Verification items for the finished model (mm, model axes). A direction names the side the tool comes from. Coordinates: 2 decimals unless noted, no trailing zeros. Order: outer loops, then holes, each group sorted by start corner. A loop starts at its lowest first (then second) coordinate and runs counter-clockwise, first axis right, second up. Notation, with made-up numbers: M 69,69 L 116,69 A21 cw 116,84 Z; hole C -26.5,70.25 d6. An arc over 180 degrees is marked long. Return JSON: item names as keys, results as strings. Group by question number.
Q1. Section check B-B, the plane x = 0. Enter the section's corners in (y, z).
Q2. Thickness scan on probe 1 along Z at (x, y) = (0, 26.5); probe 2 along Z at (x, y) = (-0.25, 63.5); probe 3 along Y at (x, z) = (3.25, 5.5). Record the ranges inside material, lowest first.
Q3. Section check D-D, the plane y = 60. Enter the section's corners in (x, z).
Q4. Section check A-A, the plane z = 0. Enter the section's corners in (x, y), then the cut area to 3 significant figures.
Q5. Mould release check, pull along X, two halves, no side actions. Record for faces 3 (the face through (0, 50.8, 0)), 4 (the face through (-2.87, 25.04, 2.64)), 5 (the face through (-1.65, 68.6, 7.44)), 6 (the face through (0, 69.85, 0)): pulls with the +X half, pulls with the -X half, needs draft (parallel to the pull), parting line crosses it, or undercut.
Q6. Section check C-C, the plane y = 18.5. Enter the section's corners in (x, z), then the cut area to 3 significant figures.
Q7. Go/stop test with flat-tipped pins: pin 1 Ø4 at (x, y) = (-4, 12) entering from -Z; pin 2 Ø3 at (x, z) = (-5.5, -0.5) entering from -Y; pin 3 Ø3 at (x, y) = (4.5, 14) entering from -Z; pin 4 Ø5 at (x, y) = (5, 41.5) entering from -Z. Record where each tip stops, or that it passes through.
Q8. Access from +Z, -Z, +X, -X, +Y, -Y to the whole of each face (thin tool, end or side, straight path). Record for faces 1 (the face through (-5.589, 33.184, 2.317)), 2 (the face through (-1, 0, -4)).
Autodesk Inventor part; units mm, degrees
ref_plane "YZ Plane" through (0, 0, 0) normal (1, 0, 0) x (0, 1, 0)
ref_plane "XZ Plane" through (0, 0, 0) normal (0, 1, 0) x (-1, 0, 0)
ref_plane "XY Plane" through (0, 0, 0) normal (0, 0, 1) x (1, 0, 0)
sketch "Sketch1" plane through (0, 0, 0) normal (0, 1, 0) x (-1, 0, 0)
  circle A0 centre (0, 0) radius 6.05
  dimension "d0" = 12.1
extrude "Extrusion1" add sketch "Sketch1" along normal blind 69.85
sketch "Sketch2" plane through (0, 69.85, 0) normal (0, 1, 0) x (1, 0, 0)
  circle A0 centre (0, 0) radius 6.7945
  circle A1 centre (0, 0) radius 7.62
  dimension "d3" = 15.24
extrude "Extrusion2" add sketch "Sketch2" against normal blind 2.54 contours A0 | A1
sketch "Sketch3" plane through (0, 0, 0) normal (0, -1, 0) x (1, 0, 0)
  circle A0 centre (0, 0) radius 3.9
  dimension "d6" = 7.8
extrude "Extrusion3" cut sketch "Sketch3" against normal blind 50.8
properties part number "Press_Head"
Numbers:
{
 "1": {"outline": "M 0,-6.05 L 67.31,-6.05 L 67.31,-7.62 L 69.85,-7.62 L 69.85,7.62 L 67.31,7.62 L 67.31,6.05 L 0,6.05 L 0,3.9 L 50.8,3.9 L 50.8,-3.9 L 0,-3.9 Z"},
 "2": {"probe 1": "z = -6.05 to -3.9, 3.9 to 6.05", "probe 2": "z = -6.04 to 6.04", "probe 3": "y = 67.31 to 69.85"},
 "3": {"outline": "C 0,0 d12.1"},
 "4": {"outline": "M -7.62,67.31 L -6.05,67.31 L -6.05,0 L -3.9,0 L -3.9,50.8 L 3.9,50.8 L 3.9,0 L 6.05,0 L 6.05,67.31 L 7.62,67.31 L 7.62,69.85 L -7.62,69.85 Z", "area": "457 mm2"},
 "5": {"face 3": "undercut", "face 4": "undercut", "face 5": "parting line crosses it", "face 6": "needs draft"},
 "6": {"outline": "C 0,0 d12.1; hole C 0,0 d7.8", "area": "67.2 mm2"},
 "7": {"pin 1": "stops at z = -5.71", "pin 2": "stops at y = 0", "pin 3": "stops at z = -5.25", "pin 4": "stops at z = -5.51"},
 "8": {"face 1": "-Y", "face 2": "+Z, -Z, +X, -X, -Y"}
}
